from build123d import *

# Parameters (mm, degrees)
SKETCH_1_R             = 6
EXTRUDE_1_DEPTH        = 3
SKETCH_2_R             = 6
EXTRUDE_2_DEPTH        = 28
HOLE_WIZARD_M6_1_D     = 5
HOLE_WIZARD_M6_1_DEPTH = 12
HOLE_WIZARD_M6_1_TIP   = 1.502151548
SKETCH_6_R             = 3
CUT_EXTRUDE_1_DEPTH    = 10


with BuildPart() as part:
    # 草图1 → 凸台-拉伸1 (new body)
    with BuildSketch(Plane(origin=(0, 0, 0), x_dir=(1, 0, 0), z_dir=(0, 1, 0))):
        with Locations((-13.5, 0)):
            Circle(SKETCH_1_R)
        with BuildLine():
            Line((13.5, 6), (-13.5, 6))
            ThreePointArc((-13.5, 6), (-9.257359313, 4.242640687), (-7.5, 0))
            ThreePointArc((-7.5, 0), (-9.257359313, -4.242640687), (-13.5, -6))
            Line((-13.5, -6), (13.5, -6))
            ThreePointArc((13.5, -6), (7.5, 0), (13.5, 6))
        make_face()
        with Locations((13.5, 0)):
            Circle(SKETCH_1_R)
    extrude(amount=EXTRUDE_1_DEPTH)

    # 草图2 → 凸台-拉伸2 (add)
    with BuildSketch(Plane(origin=(0, 3, 0), x_dir=(1, 0, 0), z_dir=(0, 1, 0))):
        Circle(SKETCH_2_R)
    extrude(amount=EXTRUDE_2_DEPTH)

    # M6 螺纹孔1
    with Locations(Plane(origin=(0, 31, 0), x_dir=(1, 0, 0), z_dir=(0, 1, 0))):
        with Locations((0, 0)):
            Hole(HOLE_WIZARD_M6_1_D / 2, depth=HOLE_WIZARD_M6_1_DEPTH)
            with Locations((0, 0, -(HOLE_WIZARD_M6_1_DEPTH + HOLE_WIZARD_M6_1_TIP / 2))):  # 118° drill point
                Cone(0, HOLE_WIZARD_M6_1_D / 2, HOLE_WIZARD_M6_1_TIP, mode=Mode.SUBTRACT)

    # 草图6 → 切除-拉伸1 (cut)
    with BuildSketch(Plane(origin=(0, 3, 0), x_dir=(1, 0, 0), z_dir=(0, 1, 0))):
        with Locations((-13.5, 0)):
            Circle(SKETCH_6_R)
        with Locations((13.5, 0)):
            Circle(SKETCH_6_R)
    extrude(amount=-CUT_EXTRUDE_1_DEPTH, mode=Mode.SUBTRACT)


solid = part.part
Geometry: final body of the model. Coordinates: model frame, mm. A direction names the side the tool comes from. Round coordinates to 2 decimals unless told otherwise and drop trailing zeros. Loops run counter-clockwise (first coordinate to the right, second up) from the corner with the lowest first, then second, coordinate; pieces in that order, holes last. Notation, with made-up numbers: (8, 68) - (56, 68) arc R17 cw to (56, 74) - close; hole circle Ø7 at (43, -27). An arc over 180 degrees is marked (long way). Write each question's results on one line, items separated by ' | '. Start each with the question number.
1) Access query for faces 4 (the face through (0.54, 24.92, 2.44)), 5 (the face through (19.5, 1.5, 0.1)). Directions: +Z, -Z, +X, -X, +Y, -Y. A direction counts if a zero-diameter tool reaches every point of the face in a straight line with its end or side. Return the directions, or none.
2) Cut plane D-D on z = 0.75. Count the separate pieces of the cut face and the enclosed holes in it, then the cut area to 3 significant figures.
3) Mould query, pull axis X, two halves, no side actions, for faces 1 (the face through (-6, 17, 0)), 2 (the face through (-10, 3, 0)), 3 (the face through (-16.5, 1.5, -0.1)). Classes: released by +X, released by -X, zero draft, split by the parting line, or undercut.
4) Cut plane A-A on x = 14. Return loops of the section in (y, z), then the cut area to 3 significant figures.
5) First-contact query: P1, Ø1, axis at x = -10.5, z = -3, coming from the -Y side; P2, Ø5, axis at y = 13.5, z = -2, coming from the +X side; P3, Ø1.5, axis at y = 7.5, z = -2.5, coming from the +X side; P4, Ø6, axis at x = -10.5, z = 3.5, coming from the +Y side. Flat tips, straight axial feed; report the tip coordinate or a pass-through.
6) Cut plane B-B on y = 27.5. Return loops of the section in (x, z), then the cut area to 3 significant figures.
7) Line query: probe 1 along X at (y, z) = (1.55, 0); probe 2 along Z at (x, y) = (-13.5, 0.85); probe 3 along Y at (x, z) = (-14, 4.5). Output: solid intervals per line, ascending. Write a range as [from, to].
8) Cut plane C-C on x = -5. Return loops of the section in (y, z), then the cut area to 3 significant figures.
Verdict:
1) face 4: +Y | face 5: +X, +Y, -Y
2) separate pieces: 3 | enclosed holes: 0 | area: 355 mm2
3) face 1: split by the parting line | face 2: zero draft | face 3: undercut
4) outline: (0, -5.98) - (3, -5.98) - (3, -2.96) - (0, -2.96) - close; (0, 2.96) - (3, 2.96) - (3, 5.98) - (0, 5.98) - close | area: 18.1 mm2
5) P1: stops at y = 0 | P2: stops at x = 6 | P3: stops at x = 5.74 | P4: stops at y = 3
6) outline: circle Ø12 at (0, 0); hole circle Ø5 at (0, 0) | area: 93.5 mm2
7) probe 1: x = [-19.5, -16.5], [-10.5, 10.5], [16.5, 19.5] | probe 2: z = [-6, -3], [3, 6] | probe 3: y = [0, 3]
8) outline: (0, -6) - (3, -6) - (3, -3.32) - (31, -3.32) - (31, 3.32) - (3, 3.32) - (3, 6) - (0, 6) - close | area: 222 mm2
